Verification items for the finished model (mm, model axes). A direction names the side the tool comes from. Give positions to 0.01 mm unless a question says otherwise; leave off trailing zeros. Loops run counter-clockwise (first coordinate to the right, second up) from the corner with the lowest first, then second, coordinate; pieces in that order, holes last. Notation, with made-up numbers: (-16.75, 60) -> (13.25, 60) arc R26 ccw to (13.25, 79) -> close; hole circle Ø3 at (22.25, -30). An arc over 180 degrees is marked (long way). Answer in a Markdown table with one row per item. Add a question column.
Q1. Material ranges on probe 1 along Y at (x, z) = (0.25, -32); probe 2 along Z at (x, y) = (0.55, -67); probe 3 along Z at (x, y) = (11.25, -30.5), recorded low to high.
Q2. Section check B-B on x = 14.5. Enter the section's corners in (y, z), and give its area (3 significant figures).
Q3. Section check D-D on y = -15.5. Enter the section's corners in (x, z), and give its area (3 significant figures).
Q4. Section check A-A on y = 53. Enter the section's corners in (x, z), and give its area (3 significant figures).
Q5. Release check for a two-part mould opening along Y. For faces 6 (the face through (9, -1, 34)), 7 (the face through (8, 70, 0)), 8 (the face through (8, 1, -35)) record: pulls with the +Y half, pulls with the -Y half, needs draft (parallel to the pull), parting line crosses it, or undercut.
Q6. Section check C-C on z = -23. Enter the section's corners in (x, y).
Q7. Gauge pin test, flat ends, axial feed: P1, Ø0.5, axis at x = -1.5, y = -2.5, coming from the +Z side; P2, Ø0.6, axis at y = -2, z = -14.5, coming from the +X side; P3, Ø2.5, axis at x = -1.5, z = -12.5, coming from the +Y side; P4, Ø2.5, axis at y = 67, z = 32, coming from the +X side. Record the tip position at first contact, or that the pin passes through.
Q8. Set-up check for faces 1 (the face through (-1, -35, 13)), 2 (the face through (9, 1, -34)), 3 (the face through (-1, 35, 12)), 4 (the face through (0.493, -65.513, -32.195)), 5 (the face through (-3, 0, -13)): record each of +Z, -Z, +X, -X, +Y, -Y from which the full face is reachable in a straight line by a thin tool's end or side.
Autodesk Fusion 360 part; units mm, degrees
sketch "Sketch1" plane through (0, 0, 0) normal (1, 0, 0) x (0, 0, -1)
  line L0 (35, -70) -> (-35, -70)
  line L1 (-35, -70) -> (-35, 70)
  line L2 (-35, 70) -> (35, 70)
  line L3 (35, 70) -> (35, -70)
  line L4 (35, -70) -> (-35, 70) construction
  line L5 (-35, -70) -> (35, 70) construction
  dimension "d1" = 70
  dimension "d2" = 140
extrude "Extrude1" add sketch "Sketch1" along normal blind 17
shell "Shell1" thickness 1 removed faces 1 at (17, -23.3333, 11.6667)
fillet "Fillet1" radius 2 1 edges at (8.5, 70, 35)
fillet "Fillet1" radius 2 1 edges at (8.5, 70, -35)
fillet "Fillet1" radius 2 1 edges at (8.5, -70, 35)
fillet "Fillet1" radius 2 1 edges at (8.5, -70, -35)
sketch "Sketch2" plane through (0, 0, 0) normal (-1, 0, 0) x (0, 0, 1)
  arc A0 (-35, -68) -> (-33, -70) centre (-33, -68) ccw
  line L0 (-33, -70) -> (33, -70)
  arc A1 (33, -70) -> (35, -68) centre (33, -68) ccw
  line L1 (35, -68) -> (35, 68)
  arc A2 (35, 68) -> (33, 70) centre (33, 68) ccw
  line L2 (33, 70) -> (-33, 70)
  arc A3 (-33, 70) -> (-35, 68) centre (-33, 68) ccw
  line L3 (-35, 68) -> (-35, -68)
  line L4 (32, 67) -> (-32, 67)
  line L5 (-32, 67) -> (-32, -67)
  line L6 (-32, -67) -> (32, -67)
  line L7 (32, -67) -> (32, 67)
  line L8 (32, 67) -> (-32, -67) construction
  line L9 (-32, 67) -> (32, -67) construction
  circle A4 centre (-32, 67) radius 1.5
  circle A5 centre (32, 67) radius 1.5
  circle A6 centre (32, -67) radius 1.5
  circle A7 centre (-32, -67) radius 1.5
  dimension "d14" = 64
  dimension "d15" = 134
  dimension "d16" = 3
  dimension "d17" = 3
  dimension "d18" = 3
  dimension "d19" = 3
extrude "Extrude2" cut sketch "Sketch2" against normal blind 10 contours L4 L5 A4 | L4 L5 A4 | L4 L7 A5 | L4 L7 A5 | L5 L6 A7 | L5 L6 A7 | L6 L7 A6 | L6 L7 A6
sketch "Sketch3" plane through (0, 0, 0) normal (-1, 0, 0) x (0, 0, 1)
  circle A0 centre (32, -67) radius 1.5
  circle A1 centre (32, 67) radius 1.5
  circle A2 centre (-32, -67) radius 1.5
  circle A3 centre (-32, 67) radius 1.5
  arc A4 (-35, -68) -> (-33, -70) centre (-33, -68) ccw
  line L0 (-33, -70) -> (33, -70)
  arc A5 (33, -70) -> (35, -68) centre (33, -68) ccw
  line L1 (35, -68) -> (35, 68)
  arc A6 (35, 68) -> (33, 70) centre (33, 68) ccw
  line L2 (33, 70) -> (-33, 70)
  arc A7 (-33, 70) -> (-35, 68) centre (-33, 68) ccw
  line L3 (-35, 68) -> (-35, -68)
  line L4 (0, 0) -> (10, 0)
  line L5 (10, 0) -> (-10, 0)
  line L6 (-10, 0) -> (-10, 35)
  line L7 (-10, 35) -> (-15, 35)
  line L8 (-15, 35) -> (-15, -35)
  line L9 (-15, -35) -> (-10, -35)
  line L10 (-10, -35) -> (-10, 0)
  line L11 (10, 0) -> (10, 35)
  line L12 (10, 35) -> (15, 35)
  line L13 (15, 35) -> (15, -35)
  line L14 (15, -35) -> (10, -35)
  line L15 (10, -35) -> (10, 0)
extrude "Extrude3" add sketch "Sketch3" along normal blind 3 contours L11 L12 L13 L14 L15 | L6 L7 L8 L9 L10
fillet "Fillet2" radius 1 1 edges at (-3, 0, 10)
fillet "Fillet2" radius 1 1 edges at (-3, 0, 15)
fillet "Fillet3" radius 1 1 edges at (-3, 0, -10)
fillet "Fillet4" radius 1 1 edges at (-3, 0, -15)
sketch "Sketch4" plane through (0, 35, 0) normal (0, 1, 0) x (-1, 0, 0)
  arc A0 (3, -11) -> (2, -10) centre (2, -11) ccw
  line L0 (2, -10) -> (0, -10)
  line L1 (0, -10) -> (0, -15)
  line L2 (0, -15) -> (2, -15)
  line L3 (0, -10) -> (2, -10)
  line L4 (2, -15) -> (0, -15)
  arc A1 (3, -11) -> (2, -10) centre (2, -11) ccw
  line L5 (0, -10) -> (0.5, -10)
  line L6 (0, -10) -> (0, -10.5)
  line L7 (1, -10.5) -> (0, -10.5)
  line L8 (0, -15) -> (0, -14.5)
  line L9 (0, -14.5) -> (1, -14.5)
  line L10 (0, -15) -> (0, -14.5)
  line L11 (0, -10.5) -> (0, -10)
  line L12 (1, -10) -> (1, -10.5)
  line L13 (1, -14.5) -> (1, -15)
  dimension "d32" = 1
extrude "Extrude4" cut sketch "Sketch4" against normal blind 70
sketch "Sketch5" plane through (0, 35, 0) normal (0, 1, 0) x (-1, 0, 0)
  arc A0 (3, 14) -> (2, 15) centre (2, 14) ccw
  line L0 (2, 15) -> (0, 15)
  line L1 (0, 15) -> (0, 10)
  line L2 (0, 10) -> (2, 10)
  arc A1 (2, 10) -> (3, 11) centre (2, 11) ccw
  line L3 (3, 11) -> (3, 14)
  line L4 (0, 15) -> (1, 15)
  line L5 (1, 15) -> (1, 14.5)
  line L6 (1, 14.5) -> (0, 14.5)
  line L7 (0, 15) -> (0, 14.5)
  line L8 (0, 10) -> (0, 10.5)
  line L9 (1, 10.5) -> (1, 10)
  line L10 (0, 10.5) -> (1, 10.5)
  line L11 (1, 10) -> (0, 10)
extrude "Extrude5" cut sketch "Sketch5" against normal blind 70 contours L0 L1 L4 L5 L6 L7 | L1 L2 L8 L9 L10 L11
Taken from the geometry:
| question | item | result |
|---|---|---|
| 1 | probe 1 | y = -70 to -68.5, -65.5 to 65.5, 68.5 to 70 |
| 1 | probe 2 | z = -35 to -33.5, -30.5 to 30.5, 33.5 to 35 |
| 1 | probe 3 | z = -35 to -34, 34 to 35 |
| 2 | outline | (-70, -33) arc R2 ccw to (-68, -35) -> (68, -35) arc R2 ccw to (70, -33) -> (70, 33) arc R2 ccw to (68, 35) -> (-68, 35) arc R2 ccw to (-70, 33) -> close; hole (-69, -34) -> (69, -34) -> (69, 34) -> (-69, 34) -> close |
| 2 | area | 413 mm² |
| 3 | outline | (-3, -14) arc R1 ccw to (-2, -15) -> (-1, -15) -> (-1, -14.5) -> (0, -14.5) -> (0, -35) -> (17, -35) -> (17, -34) -> (1, -34) -> (1, 34) -> (17, 34) -> (17, 35) -> (0, 35) -> (0, 14.5) -> (-1, 14.5) -> (-1, 15) -> (-2, 15) arc R1 ccw to (-3, 14) -> (-3, 11) arc R1 ccw to (-2, 10) -> (-1, 10) -> (-1, 10.5) -> (0, 10.5) -> (0, -10.5) -> (-1, -10.5) -> (-1, -10) -> (-2, -10) arc R1 ccw to (-3, -11) -> close |
| 3 | area | 129 mm² |
| 4 | outline | (0, -35) -> (17, -35) -> (17, -34) -> (1, -34) -> (1, 34) -> (17, 34) -> (17, 35) -> (0, 35) -> close |
| 4 | area | 102 mm² |
| 5 | face 6 | undercut |
| 5 | face 7 | pulls with the +Y half |
| 5 | face 8 | needs draft |
| 6 | outline | (0, -70) -> (17, -70) -> (17, -69) -> (1, -69) -> (1, 69) -> (17, 69) -> (17, 70) -> (0, 70) -> close |
| 7 | P1 | stops at z = 15 |
| 7 | P2 | stops at x = 1 |
| 7 | P3 | stops at y = 35 |
| 7 | P4 | passes through |
| 8 | face 1 | +Z, -Z, -X, -Y |
| 8 | face 2 | +X |
| 8 | face 3 | +Z, -Z, -X, +Y |
| 8 | face 4 | +X, -X |
| 8 | face 5 | +Z, -Z, -X, +Y, -Y |
